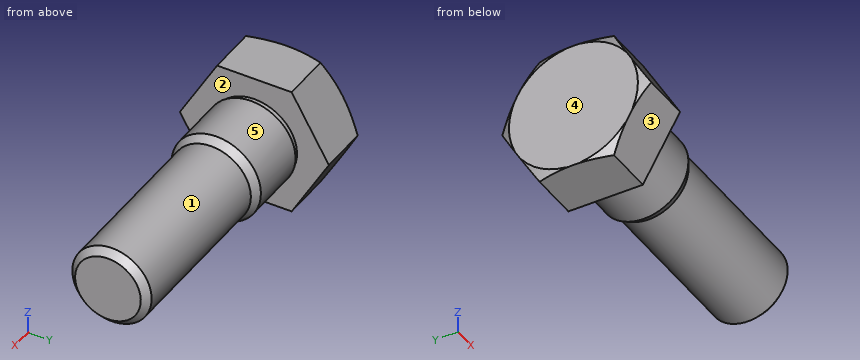
from build123d import *

# Parameters (mm, degrees)
BASEHEAD_DEPTH = 5.5


with BuildPart() as part:
    # BaseHeadSke → BaseHead (new body)
    with BuildSketch(Plane(origin=(0, 0, 0), x_dir=(0, 0, -1), z_dir=(1, 0, 0))):
        Polygon((0, 7.505553499), (-6.5, 3.75277675), (-6.5, -3.75277675), (0, -7.505553499), (6.5, -3.75277675), (6.5, 3.75277675), align=None)
    extrude(amount=BASEHEAD_DEPTH)

    # HeadChamferSke → HeadChamfer (revolve, cut)
    with BuildSketch(Plane.XY):
        Polygon((0, 7.505553499), (0, 6.5), (0.580556584, 7.505553499), align=None)
    revolve(axis=Axis((0, 0, 0), (1, 0, 0)), mode=Mode.SUBTRACT)

    # BodySke → BaseBody (revolve)
    with BuildSketch(Plane.XY, mode=Mode.PRIVATE) as basebody_sk:
        Polygon((5.5, 4.3), (6.1, 4.3), (6.1, 4.5), (12.008974596, 4.5), (12.875, 4), (29.8095, 4), (30.5, 3.3095), (30.5, 0), (5.5, 0), align=None)
    revolve(basebody_sk.sketch.rotate(Axis((0, 0, 0), (1, 0, 0)), 90), axis=Axis((0, 0, 0), (1, 0, 0)))


solid = part.part
The model under review builds one solid part; all positions refer to its coordinate system, in mm. Face numbers are marked on the shaded views. A direction names the side the tool comes from. Round coordinates to 2 decimals unless told otherwise and drop trailing zeros. Loops run counter-clockwise (first coordinate to the right, second up) from the corner with the lowest first, then second, coordinate; pieces in that order, holes last. Notation, with made-up numbers: (24, -12.5) -> (63, -12.5) arc R17 cw to (63, 9.5) -> close; hole circle Ø5 at (-15.5, 17). An arc over 180 degrees is marked (long way). Return JSON: item names as keys, results as strings.
(1) Add section A-A on x = 7. Write out the cut boundary in (y, z).
Solved:
{"outline": "circle Ø9 at (0, 0)"}
(2) For the marked faces 4 and 5, list the 3-axis set-ups (+Z, -Z, +X, -X, +Y, -Y) from which the entire face can be reached by the end or side of a thin tool; tool diameter is ignored.
Solved:
{"face 4": "+Z, -Z, -X, +Y, -Y", "face 5": "+X"}
(3) The part is to be moulded in two halves that separate along Y. For the marked faces 1, 2 and 3, say which applies: released by +Y, released by -Y, zero draft, split by the parting line, or undercut.
Solved:
{"face 1": "split by the parting line", "face 2": "zero draft", "face 3": "released by -Y"}
(4) Add section B-B on x = 14.5. Write out the cut boundary in (y, z).
Solved:
{"outline": "circle Ø8 at (0, 0)"}
(5) For pin 1 (4 mm diameter, centred on x = 20, z = 2.5, fed in from -Y); pin 2 (6 mm diameter, centred on x = 13.5, z = 3, fed in from -Y); pin 3 (3 mm diameter, centred on x = 20.5, y = -1.5, fed in from -Z), all flat-tipped, find the tip position at first contact; note any pin that passes through.
Solved:
{"pin 1": "y = -3.97", "pin 2": "y = -4.48", "pin 3": "z = -4"}
(6) For line 1 (X direction, y = 4.75, z = -1); line 2 (X direction, y = 4.25, z = 1.25); line 3 (Z direction, x = 27, y = -1), list the stretches that pass through material, from the lowest coordinate up.
Solved:
{"line 1": "0 to 5.5", "line 2": "0 to 5.5, 6.1 to 12.13", "line 3": "-3.87 to 3.87"}
